from build123d import *

# Parameters (mm, degrees)
BOSS_EXTRUDE1_DEPTH = 6.35


with BuildPart() as part:
    # Sketch1 → Boss-Extrude1 (new body)
    with BuildSketch(Plane(origin=(0, 0, 0), x_dir=(1, 0, 0), z_dir=(0, 1, 0))):
        with BuildLine():
            Line((130.67527858, 150.087360224), (156.07527858, 150.087360224))
            Line((156.07527858, 150.087360224), (156.07527858, 73.887360224))
            Line((156.07527858, 73.887360224), (130.67527858, 73.887360224))
            ThreePointArc((130.67527858, 73.887360224), (107.297701698, 30.934915456), (69.423507078, 0))
            Line((69.423507078, 0), (69.423507078, -76.2))
            ThreePointArc((69.423507078, -76.2), (107.297701698, -107.134915456), (130.67527858, -150.087360224))
            Line((130.67527858, -150.087360224), (156.07527858, -150.087360224))
            Line((156.07527858, -150.087360224), (156.07527858, -226.287360224))
            Line((156.07527858, -226.287360224), (130.67527858, -226.287360224))
            ThreePointArc((130.67527858, -226.287360224), (9.525, -315.187360224), (-111.62527858, -226.287360224))
            Line((-111.62527858, -226.287360224), (-137.02527858, -226.287360224))
            Line((-137.02527858, -226.287360224), (-137.02527858, -150.087360224))
            Line((-137.02527858, -150.087360224), (-111.62527858, -150.087360224))
            ThreePointArc((-111.62527858, -150.087360224), (-88.247701698, -107.134915456), (-50.373507078, -76.2))
            Line((-50.373507078, -76.2), (-50.373507078, 0))
            ThreePointArc((-50.373507078, 0), (-88.247701698, 30.934915456), (-111.62527858, 73.887360224))
            Line((-111.62527858, 73.887360224), (-137.02527858, 73.887360224))
            Line((-137.02527858, 73.887360224), (-137.02527858, 150.087360224))
            Line((-137.02527858, 150.087360224), (-111.62527858, 150.087360224))
            ThreePointArc((-111.62527858, 150.087360224), (9.525, 238.987360224), (130.67527858, 150.087360224))
        make_face()
        with BuildLine():
            Line((0, 0), (19.05, 0))
            Line((19.05, 0), (19.05, 15.24))
            Line((19.05, 15.24), (31.75, 15.24))
            Line((31.75, 15.24), (31.75, 6.35))
            ThreePointArc((31.75, 6.35), (9.525, 219.937360224), (-12.7, 6.35))
            Line((-12.7, 6.35), (-12.7, 15.24))
            Line((-12.7, 15.24), (0, 15.24))
            Line((0, 15.24), (0, 0))
        make_face(mode=Mode.SUBTRACT)
        with BuildLine():
            Line((0, -76.2), (19.05, -76.2))
            Line((19.05, -76.2), (19.05, -91.44))
            Line((19.05, -91.44), (31.75, -91.44))
            Line((31.75, -91.44), (31.75, -82.55))
            ThreePointArc((31.75, -82.55), (9.525, -296.137360224), (-12.7, -82.55))
            Line((-12.7, -82.55), (-12.7, -91.44))
            Line((-12.7, -91.44), (0, -91.44))
            Line((0, -91.44), (0, -76.2))
        make_face(mode=Mode.SUBTRACT)
    extrude(amount=BOSS_EXTRUDE1_DEPTH)


solid = part.part
Source: CAD feature listing. Evaluate the final solid. Frame: model axes, mm. A direction names the side the tool comes from. Round coordinates to 2 decimals unless told otherwise and drop trailing zeros. Loops run counter-clockwise (first coordinate to the right, second up) from the corner with the lowest first, then second, coordinate; pieces in that order, holes last. Notation, with made-up numbers: (34.25, -11) - (39.25, -11) arc R15 cw to (39.25, 2) - close; hole circle Ø2 at (65, 30.25). An arc over 180 degrees is marked (long way). Write item = value, one per line. Start each with the question number.
(1) Pin query (flat end, axial travel): pin 1 (3 mm diameter, centred on x = 23.5, y = 4.5, fed in from +Z); pin 2 (3 mm diameter, centred on y = 3.5, z = -10, fed in from +X); pin 3 (3 mm diameter, centred on y = 3, z = 83, fed in from +X). Return the tip coordinate at first contact, or that it passes through.
(2) Section query C-C, the plane z = -93. Output: boundary loops of the cut face in (x, y).
(3) Section query A-A, the plane x = 63.5. Output: boundary loops of the cut face in (y, z), plus the area to 3 significant figures.
(4) Pull-direction query (X, two-part tool) for faces 1 (the face through (11.776, 3.131, 315.167)), 2 (the face through (107.74, 3.13, -31.47)), 3 (the face through (-87.8, 3.1, -30.4)), 4 (the face through (13.958, 3.131, -219.846)); classes: +X half, -X half, draft (parallel to the pull), parting line (faces both ways), or undercut.
(5) Section query B-B, the plane x = -67. Output: boundary loops of the cut face in (y, z), plus the area to 4 significant figures.
(6) Section query D-D, the plane y = 4. State how many separate pieces and enclosed holes the cut face has, plus the area to 3 significant figures.
(7) Set-up query: faces 5 (the face through (106.86, 3.13, 106.61)), 6 (the face through (10, 0, 37)), 7 (the face through (-88.69, 3.13, 107.67)). Return all of +Z, -Z, +X, -X, +Y, -Y with unobstructed straight access to the full face (end or side cutting, diameter ignored); none if empty.
(8) Ray query, line 1 along Z through (x, y) = (6, 1.25); line 2 along Z through (x, y) = (-75, 0.75); line 3 along Z through (x, y) = (-24.5, 5.25). Return the intervals inside material, ascending. Write a range as from..to.
Conclusion:
q1.pin_1 = 314.57
q1.pin_2 = 87.19
q1.pin_3 = 82.86
q2.outline = (-137.03, 0) - (-96.74, 0) - (-96.74, 6.35) - (-137.03, 6.35) - close; (115.79, 0) - (156.08, 0) - (156.08, 6.35) - (115.79, 6.35) - close
q3.outline = (0, -226.95) - (6.35, -226.95) - (6.35, -205.47) - (0, -205.47) - close; (0, -18.5) - (6.35, -18.5) - (6.35, 94.7) - (0, 94.7) - close; (0, 281.67) - (6.35, 281.67) - (6.35, 303.15) - (0, 303.15) - close
q3.area = 992 mm2
q4.face_1 = parting line
q4.face_2 = +X half
q4.face_3 = -X half
q4.face_4 = undercut
q5.outline = (0, -213.34) - (6.35, -213.34) - (6.35, -188.13) - (0, -188.13) - close; (0, -35.85) - (6.35, -35.85) - (6.35, -10.63) - (0, -10.63) - close; (0, 86.83) - (6.35, 86.83) - (6.35, 112.05) - (0, 112.05) - close; (0, 264.33) - (6.35, 264.33) - (6.35, 289.54) - (0, 289.54) - close
q5.area = 640.5 mm2
q6.separate_pieces = 1
q6.enclosed_holes = 2
q6.area = 41,700 mm2
q7.face_5 = +X, +Y, -Y
q7.face_6 = +Z, -Z, +X, -X, -Y
q7.face_7 = -X, +Y, -Y
q8.line_1 = -238.94..-219.88, 0..76.2, 296.08..315.14
q8.line_2 = -206.77..-179.13, -44.84..-17.2, 93.4..121.04, 255.33..282.97
q8.line_3 = -234.34..-214.43, -9.54..85.74, 290.63..310.54
